from build123d import *


with BuildPart() as f1:
    # F0 (on Front) → F1 (revolve)
    with BuildSketch(Plane.XZ):
        with BuildLine():
            Line((0, -9.75), (0, -2.75))
            Line((0, -2.75), (0, 2.75))
            ThreePointArc((0, 2.75), (-1.944544, 1.944544), (-2.75, 0))
            Line((-2.75, 0), (-2.75, -3.224587))
            ThreePointArc((-2.75, -3.224587), (-2.459809, -4.511807), (-1.645377, -5.55))
            Line((-1.645377, -5.55), (-1.584104, -5.599942))
            ThreePointArc((-1.584104, -5.599942), (-1.448365, -5.772975), (-1.4, -5.987511))
            Line((-1.4, -5.987511), (-1.4, -7.992691))
            ThreePointArc((-1.4, -7.992691), (-1.344584, -8.221482), (-1.190619, -8.399558))
            Line((-1.190619, -8.399558), (-0.909381, -8.600442))
            ThreePointArc((-0.909381, -8.600442), (-0.755416, -8.778518), (-0.7, -9.007309))
            Line((-0.7, -9.007309), (-0.7, -9.25))
            ThreePointArc((-0.7, -9.25), (-0.553553, -9.603553), (-0.2, -9.75))
            Line((-0.2, -9.75), (0, -9.75))
        make_face()
    revolve(axis=Axis((0, 0, -3.5), (0, 0, 1)))


solid = f1.part
The listing builds one solid part. Answer for the finished solid, in the listing's coordinates (mm). A direction names the side the tool comes from. Give positions to 0.01 mm unless a question says otherwise; leave off trailing zeros. Write each loop counter-clockwise with the first axis right and the second up, starting at its lowest first coordinate (ties: lowest second). Pieces come first, ordered by that corner, then holes. Notation, with made-up numbers: (-30.5, 43) - (-8.5, 43) arc R28 ccw to (-8.5, 66) - close; hole circle Ø7 at (7, 43.5). An arc over 180 degrees is marked (long way). Use a Markdown table: item, result.
1. Section A-A on z = -7 is taken. Write down the section's boundary in (x, y).
Values follow:
| item | result |
|---|---|
| outline | circle Ø2.8 at (0, 0) |
2. Section B-B on z = -1.25 is taken. Write down the section's boundary in (x, y), plus the area to 3 significant figures.
Values follow:
| item | result |
|---|---|
| outline | circle Ø5.5 at (0, 0) |
| area | 23.8 mm² |
3. Each of these flat-tipped pins is pushed along its axis until it touches: P1, Ø2, axis at x = -0.5, y = -1.5, coming from the +Z side; P2, Ø1, axis at x = 1.5, y = 1, coming from the +Z side; P3, Ø3, axis at x = 0, y = -0.5, coming from the -Z side; P4, Ø2, axis at x = 2, y = 1.5, coming from the +Z side. Where does it stop, or does it pass through?
Values follow:
| item | result |
|---|---|
| P1 | stops at z = 2.69 |
| P2 | stops at z = 2.42 |
| P3 | stops at z = -9.75 |
| P4 | stops at z = 2.3 |
4. A tool of negligible diameter and unlimited length cuts with its end or side. For faces 1 (the cylindrical face through (1.4, -0.06, -7)), 2 (the cylindrical face through (0.596, 2.685, -1.635)), from which of +Z, -Z, +X, -X, +Y, -Y can it reach the whole face along a straight path? Write none if from no direction.
Values follow:
| item | result |
|---|---|
| face 1 | -Z |
| face 2 | +Z, -Z |
5. Find the intervals of material crossed by probe 1 along X at (y, z) = (-0.7, -6.25); probe 2 along X at (y, z) = (-1.8, 0.75); probe 3 along Z at (x, y) = (1.5, 0.95), in increasing order. Write a range as from..to.
Values follow:
| item | result |
|---|---|
| probe 1 | x = -1.21..1.21 |
| probe 2 | x = -1.94..1.94 |
| probe 3 | z = -5.44..2.1 |
